Source: CAD feature listing. Evaluate the final solid. Frame: model axes, mm. A direction names the side the tool comes from. Give positions to 0.01 mm unless a question says otherwise; leave off trailing zeros. Order: outer loops, then holes, each group sorted by start corner. A loop starts at its lowest first (then second) coordinate and runs counter-clockwise, first axis right, second up. Notation, with made-up numbers: (46.25, -27) - (98.25, -27) arc R32 ccw to (98.25, -1) - close; hole circle Ø6 at (-12, 54.25). An arc over 180 degrees is marked (long way). Use CSV: the item, a comma, the result in double quotes.
```python
from build123d import *

# Parameters (mm, degrees)
BOSS_EXTRU_1_DEPTH = 1.6
ESQUISSE2_W        = 165
ESQUISSE2_H        = 100
BOSS_EXTRU_2_DEPTH = 7


with BuildPart() as part:
    # Esquisse1 → Boss.-Extru.1 (new body)
    with BuildSketch(Plane.XY):
        with BuildLine():
            Line((-82.5, 53.5), (-82.5, 55.65))
            ThreePointArc((-82.5, 55.65), (-78, 60.15), (-73.5, 55.65))
            Line((-73.5, 55.65), (-73.5, 53.5))
            Line((-73.5, 53.5), (73.5, 53.5))
            Line((73.5, 53.5), (73.5, 55.65))
            ThreePointArc((73.5, 55.65), (78, 60.15), (82.5, 55.65))
            Line((82.5, 55.65), (82.5, 53.5))
            Line((82.5, 53.5), (82.5, -53.5))
            Line((82.5, -53.5), (82.5, -55.65))
            ThreePointArc((82.5, -55.65), (78, -60.15), (73.5, -55.65))
            Line((73.5, -55.65), (73.5, -53.5))
            Line((73.5, -53.5), (-73.5, -53.5))
            Line((-73.5, -53.5), (-73.5, -55.65))
            ThreePointArc((-73.5, -55.65), (-78, -60.15), (-82.5, -55.65))
            Line((-82.5, -55.65), (-82.5, -53.5))
            Line((-82.5, -53.5), (-82.5, 53.5))
        make_face()
    extrude(amount=BOSS_EXTRU_1_DEPTH)

    # Esquisse2 → Boss.-Extru.2 (add)
    with BuildSketch(Plane.XY.offset(1.6)):
        with Locations((0, 1.5)):
            Rectangle(ESQUISSE2_W, ESQUISSE2_H)
    extrude(amount=BOSS_EXTRU_2_DEPTH)


solid = part.part
```
Item 1: Section B-B on z = 5.5. Return the cut outline in (x, y), then the cut area to 3 significant figures.
Filled in:
outline,"(-82.5, -48.5) - (82.5, -48.5) - (82.5, 51.5) - (-82.5, 51.5) - close"
area,"16,500 mm2"
Item 2: Material intervals for line 1 (Y direction, x = -57, z = 2.25); line 2 (Y direction, x = 73, z = 1), sorted ascending. Write a range as from..to.
Filled in:
line 1,"y = -48.5..51.5"
line 2,"y = -53.5..53.5"
Item 3: Mould query, pull axis X, two halves, no side actions, for faces 1 (the flat face through (-82.5, -1, 4)), 2 (the cylindrical face through (78.1, -60.15, 0.79)), 3 (the flat face through (82.5, 1, 4)). Classes: released by +X, released by -X, zero draft, split by the parting line, or undercut.
Filled in:
face 1,"released by -X"
face 2,"undercut"
face 3,"released by +X"
Item 4: First-contact query: pin 1 (3 mm diameter, centred on x = 57.5, z = 4.5, fed in from -Y); pin 2 (9.5 mm diameter, centred on x = -37, y = -55.5, fed in from +Z); pin 3 (1.8 mm diameter, centred on x = 2, z = 1, fed in from -Y). Flat tips, straight axial feed; report the tip coordinate or a pass-through.
Filled in:
pin 1,"stops at y = -48.5"
pin 2,"stops at z = 1.6"
pin 3,"stops at y = -53.5"
Item 5: Section A-A on x = 58.5. Return the cut outline in (y, z), then the cut area to 3 significant figures.
Filled in:
outline,"(-53.5, 0) - (53.5, 0) - (53.5, 1.6) - (51.5, 1.6) - (51.5, 8.6) - (-48.5, 8.6) - (-48.5, 1.6) - (-53.5, 1.6) - close"
area,"871 mm2"
Item 6: Section C-C on x = -78. Return the cut outline in (y, z), then the cut area to 3 significant figures.
Filled in:
outline,"(-60.15, 0) - (60.15, 0) - (60.15, 1.6) - (51.5, 1.6) - (51.5, 8.6) - (-48.5, 8.6) - (-48.5, 1.6) - (-60.15, 1.6) - close"
area,"892 mm2"
Item 7: Set-up query: faces 4 (the cylindrical face through (-77.9, -60.15, 0.79)), 5 (the flat face through (1, -52, 1.6)), 6 (the flat face through (-1, 51.5, 5)). Return all of +Z, -Z, +X, -X, +Y, -Y with unobstructed straight access to the full face (end or side cutting, diameter ignored); none if empty.
Filled in:
face 4,"+Z, -Z, -Y"
face 5,"+Z, +X, -X, -Y"
face 6,"+Z, +X, -X, +Y"
